from build123d import *

# Parameters (mm, degrees)
IZIM1_W                     = 300
IZIM1_H                     = 180
IZIM1_R                     = 10
Y_KSEKLIK_EKSTR_ZYON1_DEPTH = 10
IZIM3_W                     = 120
IZIM3_H                     = 10
Y_KSEKLIK_EKSTR_ZYON2_DEPTH = 10
IZIM4_W                     = 20
IZIM4_H                     = 10
KES_EKSTR_ZYON1_DEPTH       = 10


with BuildPart() as part:
    # Çizim1 → Yükseklik-Ekstrüzyon1 (new body)
    with BuildSketch(Plane.XY):
        Rectangle(IZIM1_W, IZIM1_H)
        with Locations((-70, 10)):
            Circle(IZIM1_R, mode=Mode.SUBTRACT)
        with BuildLine():
            Line((100, -12.5), (40, -12.5))
            ThreePointArc((40, -12.5), (17.5, 10), (40, 32.5))
            Line((40, 32.5), (100, 32.5))
            ThreePointArc((100, 32.5), (122.5, 10), (100, -12.5))
        make_face(mode=Mode.SUBTRACT)
        with BuildLine():
            Line((100, 42.9), (40, 42.9))
            ThreePointArc((40, 42.9), (37.9, 45), (40, 47.1))
            Line((40, 47.1), (100, 47.1))
            ThreePointArc((100, 47.1), (102.1, 45), (100, 42.9))
        make_face(mode=Mode.SUBTRACT)
        with BuildLine():
            Line((100, -27.1), (40, -27.1))
            ThreePointArc((40, -27.1), (37.9, -25), (40, -22.9))
            Line((40, -22.9), (100, -22.9))
            ThreePointArc((100, -22.9), (102.1, -25), (100, -27.1))
        make_face(mode=Mode.SUBTRACT)
    extrude(amount=Y_KSEKLIK_EKSTR_ZYON1_DEPTH)

    # Çizim3 → Yükseklik-Ekstrüzyon2 (add)
    with BuildSketch(Plane(origin=(0, 90, 0), x_dir=(1, 0, 0), z_dir=(0, 1, 0))):
        with Locations((70, -5)):
            Rectangle(IZIM3_W, IZIM3_H)
        with Locations((-70, -5)):
            Rectangle(IZIM3_W, IZIM3_H)
    extrude(amount=Y_KSEKLIK_EKSTR_ZYON2_DEPTH)

    # Çizim4 → Kes-Ekstrüzyon1 (cut)
    with BuildSketch(Plane.XZ.offset(90)):
        with Locations((140, 5)):
            Rectangle(IZIM4_W, IZIM4_H)
        with Locations((0, 5)):
            Rectangle(IZIM4_W, IZIM4_H)
        with Locations((-140, 5)):
            Rectangle(IZIM4_W, IZIM4_H)
    extrude(amount=-KES_EKSTR_ZYON1_DEPTH, mode=Mode.SUBTRACT)


solid = part.part
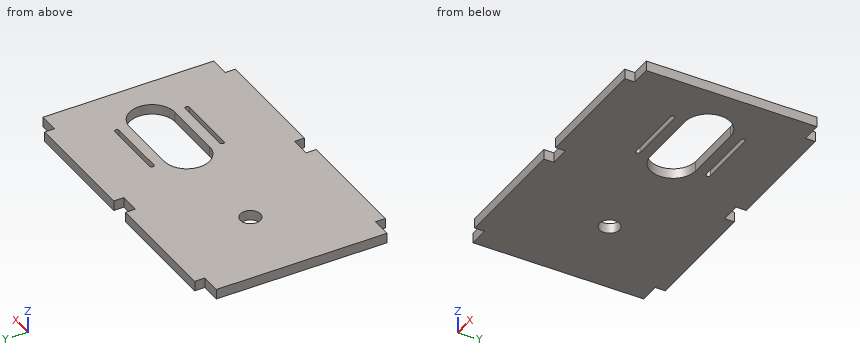
Input: part model. Units: mm. Frame: model coordinates. Give positions to 0.01 mm unless a question says otherwise; leave off trailing zeros. Order: outer loops, then holes, each group sorted by start corner. A loop starts at its lowest first (then second) coordinate and runs counter-clockwise, first axis right, second up. Notation, with made-up numbers: (28.25, 20.25) - (65.25, 20.25) arc R36 cw to (65.25, 57.25) - close; hole circle Ø3 at (-14, 61.5). An arc over 180 degrees is marked (long way). Write each question's results on one line, items separated by ' | '.
Item 1: Section C-C (y = 10). Return loops of the section in (x, z), and give its area (3 significant figures).
A:
outline: (-150, 0) - (-80, 0) - (-80, 10) - (-150, 10) - close; (-60, 0) - (17.5, 0) - (17.5, 10) - (-60, 10) - close; (122.5, 0) - (150, 0) - (150, 10) - (122.5, 10) - close | area: 1,750 mm^2
Item 2: Section D-D (x = -70). Return loops of the section in (y, z), and give its area (3 significant figures).
A:
outline: (-90, 0) - (0, 0) - (0, 10) - (-90, 10) - close; (20, 0) - (100, 0) - (100, 10) - (20, 10) - close | area: 1,700 mm^2
Item 3: Contact query for flat-ended pins moving along their axis: pin 1 Ø5 at (y, z) = (-85.5, 5) entering from -X; pin 2 Ø3 at (y, z) = (97.5, 4.5) entering from +X. Output: stop coordinate, or through.
A:
pin 1: stops at x = -130 | pin 2: stops at x = 130
Item 4: Section A-A (x = 86). Return loops of the section in (y, z).
A:
outline: (-90, 0) - (-27.1, 0) - (-27.1, 10) - (-90, 10) - close; (-22.9, 0) - (-12.5, 0) - (-12.5, 10) - (-22.9, 10) - close; (32.5, 0) - (42.9, 0) - (42.9, 10) - (32.5, 10) - close; (47.1, 0) - (100, 0) - (100, 10) - (47.1, 10) - close
Item 5: Section B-B (z = 8.5). Give the number of separate pieces and of enclosed holes in the cut face, and give its area (3 significant figures).
A:
separate pieces: 1 | enclosed holes: 4 | area: 50,700 mm^2
Item 6: Material intervals for line 1 along Y through (x, z) = (67, 5.5); line 2 along Y through (x, z) = (-70, 5.75); line 3 along X through (y, z) = (2, 7), sorted ascending.
A:
line 1: y = -90 to -27.1, -22.9 to -12.5, 32.5 to 42.9, 47.1 to 100 | line 2: y = -90 to 0, 20 to 100 | line 3: x = -150 to -76, -64 to 18.97, 121.03 to 150
